```python
from build123d import *

# Parameters (mm, degrees)
F1_DEPTH = 114.3
F3_D     = 19.05
F3_DEPTH = 50.8
F3_TIP   = 5.7231973962


with BuildPart() as f1:
    # F0 (on Right) → F1 (new body)
    with BuildSketch(Plane.YZ):
        Polygon((127, 0), (0, 0), (-57.6322190464, -42.119871825), (-57.6322190464, -115.8806011081), (127, -115.8806011081), align=None)
    extrude(amount=F1_DEPTH)

    # F3
    with Locations(Plane(origin=(0, 0, 0), x_dir=(1, 0, 0), z_dir=(0, -0.5900532948, 0.8073642977))):
        with Locations((74.9021172523, -33.4962010384), (26.8135797232, -33.4962010384)):
            Hole(F3_D / 2, depth=F3_DEPTH)
            with Locations((0, 0, -(F3_DEPTH + F3_TIP / 2))):  # 118° drill point
                Cone(0, F3_D / 2, F3_TIP, mode=Mode.SUBTRACT)


solid = f1.part
```
Here's how the part is built. I have some questions about the finished solid (model axes, mm). A direction names the side the tool comes from. Give positions to 0.01 mm unless a question says otherwise; leave off trailing zeros. Order: outer loops, then holes, each group sorted by start corner. A loop starts at its lowest first (then second) coordinate and runs counter-clockwise, first axis right, second up. Notation, with made-up numbers: M -27.5,88 L -11.5,88 A15 cw -11.5,117 Z; hole C 77,-3 d1. An arc over 180 degrees is marked long. Use a Markdown table: item, result. Add a question column.
1. On a 3-axis mill with a long thin cutter (end or side, diameter ignored), from which of +Z, -Z, +X, -X, +Y, -Y can I reach the whole of each face in a straight line? I mean faces 1 (the conical face through (76.43, 5.21, -64.97)), 2 (the flat face through (114.3, 33, -57)). Say none if no direction works.
2. Suppose I cut it at B-B (y = -37.5). List the corners of the cut face in (x, z) for me.
3. I need wall thicknesses on probe 1 along Y at (x, z) = (30, -41); probe 2 along Y at (x, z) = (31.5, -64); probe 3 along Y at (x, z) = (9, -13). Which ranges of each line are inside material? Lowest first, please. Write a range as from..to.
4. Suppose I cut it at C-C (z = -34.5). Give the number of separate pieces and of enclosed holes in the cut face, and give its area (3 significant figures).
5. Suppose I cut it at A-A (x = 60.5). List the corners of the cut face in (y, z) for me.
6. If we mould it in two halves opening along Y, with no side actions, what happens to faces 3 (the cylindrical face through (18.015, -14.792, -42.711)), 4 (the flat face through (56, 33, -115.881)), 5 (the flat face through (56, 127, -59))? For each: +Y half, -Y half, draft (parallel to the pull), parting line (faces both ways), or undercut.
Results list:
| question | item | result |
|---|---|---|
| 1 | face 1 | none |
| 1 | face 2 | +Z, -Z, +X, +Y, -Y |
| 2 | outline | M 0,-115.88 L 114.3,-115.88 L 114.3,-27.41 L 0,-27.41 Z |
| 3 | probe 1 | y = -56.1..-22.64, -0.41..127 |
| 3 | probe 2 | y = -57.63..-4.99, 3.13..127 |
| 3 | probe 3 | y = -17.79..127 |
| 4 | separate pieces | 1 |
| 4 | enclosed holes | 2 |
| 4 | area | 19,200 mm² |
| 5 | outline | M -57.63,-115.88 L 127,-115.88 L 127,0 L 0,0 L -57.63,-42.12 Z |
| 6 | face 3 | undercut |
| 6 | face 4 | draft |
| 6 | face 5 | +Y half |
